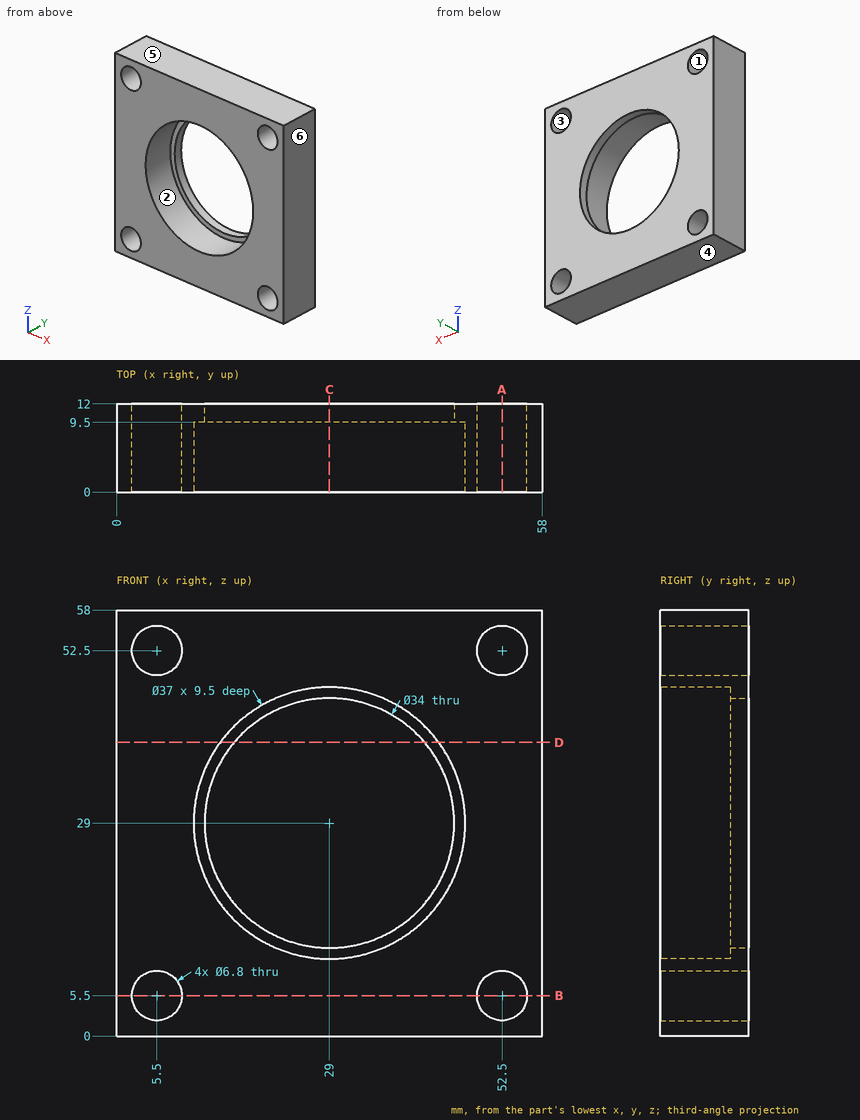
Input: dimensioned drawing with shaded views. Units: mm. Origin: part minimum x, y, z. A direction names the side the tool comes from. Coordinates: 2 decimals unless noted, no trailing zeros. Loops run counter-clockwise (first coordinate to the right, second up) from the corner with the lowest first, then second, coordinate; pieces in that order, holes last.
Q1. Section C-C, the plane x = 29. Return the cut outline in (y, z).
Results are:
outline: (0, 0) - (12, 0) - (12, 12) - (9.5, 12) - (9.5, 10.5) - (0, 10.5) - close; (0, 47.5) - (9.5, 47.5) - (9.5, 46) - (12, 46) - (12, 58) - (0, 58) - close
Q2. Contact query for a flat-ended pin moving along its axis: pin 1 (4 mm diameter, centred on x = 52.5, z = 5.5, fed in from -Y). Output: stop coordinate, or through.
Results are:
pin 1: passes through
Q3. Section B-B, the plane z = 5.5. Return the cut outline in (x, y).
Results are:
outline: (0, 0) - (2.1, 0) - (2.1, 12) - (0, 12) - close; (8.9, 0) - (49.1, 0) - (49.1, 12) - (8.9, 12) - close; (55.9, 0) - (58, 0) - (58, 12) - (55.9, 12) - close
Q4. Line query: line 1 along Z through (x, y) = (52.5, 8.25); line 2 along X through (y, z) = (5, 51); line 3 along Z through (x, y) = (29, 11). Output: solid intervals per line, ascending.
Results are:
line 1: z = 0 to 2.1, 8.9 to 49.1, 55.9 to 58
line 2: x = 0 to 2.45, 8.55 to 49.45, 55.55 to 58
line 3: z = 0 to 12, 46 to 58
Q5. Mould query, pull axis Z, two halves, no side actions, for the marked faces 3, 4, 5 and 6. Classes: +Z half, -Z half, draft (parallel to the pull), parting line (faces both ways), or undercut.
Results are:
face 3: undercut
face 4: -Z half
face 5: +Z half
face 6: draft
Q6. Section D-D, the plane z = 40. Return the cut outline in (x, y).
Results are:
outline: (0, 0) - (14.13, 0) - (14.13, 9.5) - (16.04, 9.5) - (16.04, 12) - (0, 12) - close; (41.96, 9.5) - (43.87, 9.5) - (43.87, 0) - (58, 0) - (58, 12) - (41.96, 12) - close
Q7. Section A-A, the plane x = 52.5. Return the cut outline in (y, z), and give its area (3 significant figures).
Results are:
outline: (0, 0) - (12, 0) - (12, 2.1) - (0, 2.1) - close; (0, 8.9) - (12, 8.9) - (12, 49.1) - (0, 49.1) - close; (0, 55.9) - (12, 55.9) - (12, 58) - (0, 58) - close
area: 533 mm2
Q8. Set-up query: the marked faces 1 and 2. Return all of +Z, -Z, +X, -X, +Y, -Y with unobstructed straight access to the full face (end or side cutting, diameter ignored); none if empty.
Results are:
face 1: +Y, -Y
face 2: -Y
